from build123d import *

# Parameters (mm, degrees)
F0_W      = 55
F0_H      = 160
F1_DEPTH  = 20
F2_W      = 55
F2_H      = 160
F3_DEPTH  = 155
F4_R      = 2.5
F5_DEPTH  = 5
F6_W      = 7
F6_H      = 39
F7_DEPTH  = 8
F8_W      = 14.6
F8_H      = 102.5
F8_W_2    = 14
F8_H_2    = 88.35
F8_W_3    = 20.1
F8_H_3    = 11.3
F8_W_4    = 39
F8_H_4    = 13
F8_R      = 2.25
F9_DEPTH  = 2
F10_W     = 40
F10_H     = 12
F10_H_2   = 8
F11_DEPTH = 35
F12_R     = 30
F13_DEPTH = 2


with BuildPart() as f1:
    # F0 (on Front) → F1 (new body)
    with BuildSketch(Plane.XZ):
        with Locations((27.5, 80)):
            Rectangle(F0_W, F0_H)
    extrude(amount=-F1_DEPTH)

    # F2 (on face) → F3 (join)
    with BuildSketch(Plane(origin=(0, 20, 0), x_dir=(-1, 0, 0), z_dir=(0, 1, 0))):
        with BuildLine():
            Line((3, 160), (0, 160))
            Line((0, 160), (0, 0))
            Line((0, 0), (27, 0))
            Line((27, 0), (35, 8))
            Line((35, 8), (35, 144.66))
            Line((35, 144.66), (7.131759, 149.573923))
            ThreePointArc((7.131759, 149.573923), (4.169778, 151.284023), (3, 154.497962))
            Line((3, 154.497962), (3, 160))
        make_face()
        with Locations((-27.5, 80)):
            Rectangle(F2_W, F2_H)
    extrude(amount=F3_DEPTH)

    # F4 (on face) → F5 (join)
    with BuildSketch(Plane(origin=(0, 175, 0), x_dir=(-1, 0, 0), z_dir=(0, 1, 0))):
        with BuildLine():
            Line((9, 160), (3, 160))
            Line((3, 160), (3, 154.497962))
            ThreePointArc((3, 154.497962), (4.169778, 151.284023), (7.131759, 149.573923))
            Line((7.131759, 149.573923), (14, 148.362867))
            Line((14, 148.362867), (14, 155))
            ThreePointArc((14, 155), (12.535534, 158.535534), (9, 160))
        make_face()
        with Locations((7.5, 154.5)):
            Circle(F4_R, mode=Mode.SUBTRACT)
        with BuildLine():
            Line((3, 160), (-55, 160))
            Line((-55, 160), (-55, 0))
            Line((-55, 0), (27, 0))
            Line((27, 0), (35, 8))
            Line((35, 8), (35, 144.66))
            Line((35, 144.66), (14, 148.362867))
            Line((14, 148.362867), (7.131759, 149.573923))
            ThreePointArc((7.131759, 149.573923), (4.169778, 151.284023), (3, 154.497962))
            Line((3, 154.497962), (3, 160))
        make_face()
        with Locations((7.5, 5)):
            Circle(F4_R, mode=Mode.SUBTRACT)
    extrude(amount=F5_DEPTH)

    # F6 (on face) → F7 (join)
    with BuildSketch(Plane.YZ.offset(55)):
        with Locations((35, 125.5)):
            Rectangle(F6_W, F6_H)
    extrude(amount=F7_DEPTH)

    # F8 (on face) → F9 (cut)
    with BuildSketch(Plane.XZ):
        with Locations((10.2, 54.8)):
            Rectangle(F8_W, F8_H)
        with Locations((43.3, 61.825)):
            Rectangle(F8_W_2, F8_H_2)
        with Locations((41.85, 9.2)):
            Rectangle(F8_W_3, F8_H_3)
        with Locations((24.1, 133)):
            Rectangle(F8_W_4, F8_H_4)
        with BuildLine():
            Line((11.1, 125), (6.6, 125))
            ThreePointArc((6.6, 125), (5.185786, 124.414214), (4.6, 123))
            Line((4.6, 123), (4.6, 120))
            ThreePointArc((4.6, 120), (5.185786, 118.585786), (6.6, 118))
            Line((6.6, 118), (11.1, 118))
            ThreePointArc((11.1, 118), (12.514214, 118.585786), (13.1, 120))
            Line((13.1, 120), (13.1, 123))
            ThreePointArc((13.1, 123), (12.514214, 124.414214), (11.1, 125))
        make_face()
        with BuildLine():
            ThreePointArc((15.1, 120), (15.685786, 118.585786), (17.1, 118))
            Line((17.1, 118), (21.1, 118))
            ThreePointArc((21.1, 118), (22.514214, 118.585786), (23.1, 120))
            Line((23.1, 120), (23.1, 123))
            ThreePointArc((23.1, 123), (22.514214, 124.414214), (21.1, 125))
            Line((21.1, 125), (17.1, 125))
            ThreePointArc((17.1, 125), (15.685786, 124.414214), (15.1, 123))
            Line((15.1, 123), (15.1, 120))
        make_face()
        with BuildLine():
            ThreePointArc((25.1, 120), (25.685786, 118.585786), (27.1, 118))
            Line((27.1, 118), (31.1, 118))
            ThreePointArc((31.1, 118), (32.514214, 118.585786), (33.1, 120))
            Line((33.1, 120), (33.1, 123))
            ThreePointArc((33.1, 123), (32.514214, 124.414214), (31.1, 125))
            Line((31.1, 125), (27.1, 125))
            ThreePointArc((27.1, 125), (25.685786, 124.414214), (25.1, 123))
            Line((25.1, 123), (25.1, 120))
        make_face()
        with BuildLine():
            ThreePointArc((35.1, 120), (35.685786, 118.585786), (37.1, 118))
            Line((37.1, 118), (41.6, 118))
            ThreePointArc((41.6, 118), (43.014214, 118.585786), (43.6, 120))
            Line((43.6, 120), (43.6, 123))
            ThreePointArc((43.6, 123), (43.014214, 124.414214), (41.6, 125))
            Line((41.6, 125), (37.1, 125))
            ThreePointArc((37.1, 125), (35.685786, 124.414214), (35.1, 123))
            Line((35.1, 123), (35.1, 120))
        make_face()
        with Locations((43.7, 112)):
            Circle(F8_R)
        with Locations((12.1, 112)):
            Circle(F8_R)
    extrude(amount=-F9_DEPTH, mode=Mode.SUBTRACT)

    # F10 (on face) → F11 (cut)
    with BuildSketch(Plane(origin=(-35, 0, 0), x_dir=(0, -1, 0), z_dir=(-1, 0, 0))):
        with Locations((-155, 14)):
            Rectangle(F10_W, F10_H)
        with Locations((-155, 4)):
            Rectangle(F10_W, F10_H_2)
    extrude(amount=-F11_DEPTH, mode=Mode.SUBTRACT)

    # F12 (on face) → F13 (cut)
    with BuildSketch(Plane(origin=(-35, 0, 0), x_dir=(0, -1, 0), z_dir=(-1, 0, 0))):
        with Locations((-100, 76.33)):
            Circle(F12_R)
    extrude(amount=-F13_DEPTH, mode=Mode.SUBTRACT)


solid = f1.part
Check sheet for the modelled part. Datum: model origin and axes. Units: mm. A direction names the side the tool comes from. Round coordinates to 2 decimals unless told otherwise and drop trailing zeros. Loops run counter-clockwise (first coordinate to the right, second up) from the corner with the lowest first, then second, coordinate; pieces in that order, holes last. Notation, with made-up numbers: M -28.75,-7.5 L 28.25,-7.5 A17 ccw 28.25,23.5 Z; hole C 59,19.5 d3. An arc over 180 degrees is marked long. One line per item, written item: value.
(1) Depth check by flat-ended pin: pin 1 Ø2.5 at (y, z) = (177.5, 152.5) entering from -X; pin 2 Ø10.5 at (x, z) = (-12.5, 65.5) entering from -Y; pin 3 Ø2 at (x, z) = (39, 123) entering from -Y. Enter the tip coordinate at first touch or a pass-through.
Computed values:
pin 1: stops at x = -14
pin 2: stops at y = 20
pin 3: stops at y = 2
(2) Thickness scan on line 1 (Z direction, x = -7.5, y = 176.1); line 2 (Z direction, x = -7, y = 177); line 3 (Z direction, x = 43, y = 1). Record the ranges inside material, lowest first.
Computed values:
line 1: z = 0 to 2.5, 7.5 to 152, 157 to 160
line 2: z = 0 to 2.55, 7.45 to 152.05, 156.95 to 160
line 3: z = 0 to 3.55, 14.85 to 17.65, 106 to 109.86, 114.14 to 118.57, 124.43 to 126.5, 139.5 to 160
(3) Sectioned sample at C-C, the plane z = 28.5. Record the cut outline in (x, y).
Computed values:
outline: M -35,20 L 0,20 L 0,0 L 2.9,0 L 2.9,2 L 17.5,2 L 17.5,0 L 36.3,0 L 36.3,2 L 50.3,2 L 50.3,0 L 55,0 L 55,180 L -35,180 Z
(4) Sectioned sample at D-D, the plane y = 143.5. Record the cut outline in (x, z).
Computed values:
outline: M -35,20 L 0,20 L 0,0 L 55,0 L 55,160 L -3,160 L -3,154.5 A5 cw -7.13,149.57 L -35,144.66 Z
(5) Access from +Z, -Z, +X, -X, +Y, -Y to the whole of each face (thin tool, end or side, straight path). Record for faces 4 (the face through (-34.014, 122.111, 96.605)), 5 (the face through (-10, 175, 153)), 6 (the face through (10, 2, 56)).
Computed values:
face 4: -X
face 5: +Z, -X, -Y
face 6: -Y
(6) Sectioned sample at B-B, the plane y = 100. Record the cut outline in (x, z).
Computed values:
outline: M -35,8 L -27,0 L 55,0 L 55,160 L -3,160 L -3,154.5 A5 cw -7.13,149.57 L -35,144.66 L -35,106.33 L -33,106.33 L -33,46.33 L -35,46.33 Z
(7) Sectioned sample at A-A, the plane z = 112. Record the cut outline in (x, y).
Computed values:
outline: M -35,20 L 0,20 L 0,0 L 9.85,0 L 9.85,2 L 14.35,2 L 14.35,0 L 41.45,0 L 41.45,2 L 45.95,2 L 45.95,0 L 55,0 L 55,31.5 L 63,31.5 L 63,38.5 L 55,38.5 L 55,180 L -35,180 Z
(8) Release check for a two-part mould opening along X. For faces 1 (the face through (30, 89, 160)), 2 (the face through (-31, 177, 4)), 3 (the face through (12, 2, 112)) record: +X half, -X half, draft (parallel to the pull), parting line (faces both ways), or undercut.
Computed values:
face 1: draft
face 2: -X half
face 3: undercut
